from build123d import *

# Parameters (mm, degrees)
SKETCH_1_R          = 62.5
SKETCH_1_R_2        = 40.5
SKETCH_1_R_3        = 2.25
SKETCH_1_R_4        = 1.9
EXTRUDE_1_DEPTH     = 11.5
SKETCH_2_R          = 42.625
CUT_EXTRUDE_1_DEPTH = 9.5


with BuildPart() as part:
    # 草图1 → 凸台-拉伸1 (new body)
    with BuildSketch(Plane.XY):
        Circle(SKETCH_1_R)
        Circle(SKETCH_1_R_2, mode=Mode.SUBTRACT)
        with Locations((0, -52.5)):
            Circle(SKETCH_1_R_3, mode=Mode.SUBTRACT)
        with Locations((-28.383642916, -44.165810474)):
            Circle(SKETCH_1_R_3, mode=Mode.SUBTRACT)
        with Locations((-47.755679756, -21.809288183)):
            Circle(SKETCH_1_R_3, mode=Mode.SUBTRACT)
        with Locations((-51.965625699, 7.471529009)):
            Circle(SKETCH_1_R_3, mode=Mode.SUBTRACT)
        with Locations((-39.676852654, 34.380188532)):
            Circle(SKETCH_1_R_3, mode=Mode.SUBTRACT)
        with Locations((-14.790959234, 50.373381115)):
            Circle(SKETCH_1_R_3, mode=Mode.SUBTRACT)
        with Locations((14.790959234, 50.373381115)):
            Circle(SKETCH_1_R_3, mode=Mode.SUBTRACT)
        with Locations((39.676852654, 34.380188532)):
            Circle(SKETCH_1_R_3, mode=Mode.SUBTRACT)
        with Locations((51.965625699, 7.471529009)):
            Circle(SKETCH_1_R_3, mode=Mode.SUBTRACT)
        with Locations((47.755679756, -21.809288183)):
            Circle(SKETCH_1_R_3, mode=Mode.SUBTRACT)
        with Locations((28.383642916, -44.165810474)):
            Circle(SKETCH_1_R_3, mode=Mode.SUBTRACT)
        with Locations((-44.2113501, -38.309352936)):
            Circle(SKETCH_1_R_4, mode=Mode.SUBTRACT)
        with Locations((-57.90455435, -8.325418039)):
            Circle(SKETCH_1_R_4, mode=Mode.SUBTRACT)
        with Locations((-53.213471728, 24.301778261)):
            Circle(SKETCH_1_R_4, mode=Mode.SUBTRACT)
        with Locations((-31.627487821, 49.213331671)):
            Circle(SKETCH_1_R_4, mode=Mode.SUBTRACT)
        with Locations((0, 58.5)):
            Circle(SKETCH_1_R_4, mode=Mode.SUBTRACT)
        with Locations((31.627487821, 49.213331671)):
            Circle(SKETCH_1_R_4, mode=Mode.SUBTRACT)
        with Locations((53.213471728, 24.301778261)):
            Circle(SKETCH_1_R_4, mode=Mode.SUBTRACT)
        with Locations((57.90455435, -8.325418039)):
            Circle(SKETCH_1_R_4, mode=Mode.SUBTRACT)
        with Locations((44.2113501, -38.309352936)):
            Circle(SKETCH_1_R_4, mode=Mode.SUBTRACT)
        with Locations((16.481354575, -56.130338956)):
            Circle(SKETCH_1_R_4, mode=Mode.SUBTRACT)
        with Locations((-16.481354575, -56.130338956)):
            Circle(SKETCH_1_R_4, mode=Mode.SUBTRACT)
    extrude(amount=EXTRUDE_1_DEPTH)

    # 草图2 → 切除-拉伸1 (cut)
    with BuildSketch(Plane.XY.offset(11.5)):
        Circle(SKETCH_2_R)
    extrude(amount=-CUT_EXTRUDE_1_DEPTH, mode=Mode.SUBTRACT)


solid = part.part
Check sheet for the modelled part. Datum: model origin and axes. Units: mm. A direction names the side the tool comes from. Coordinates: 2 decimals unless noted, no trailing zeros. Write each loop counter-clockwise with the first axis right and the second up, starting at its lowest first coordinate (ties: lowest second). Pieces come first, ordered by that corner, then holes.
Item 1: Depth check by flat-ended pin: pin 1 Ø3 at (x, y) = (-44.21, -38.31) entering from -Z; pin 2 Ø3 at (y, z) = (3, 3) entering from +X; pin 3 Ø5 at (x, z) = (-49, 2.5) entering from +Y; pin 4 Ø5 at (x, z) = (11.5, 8.5) entering from +Y. Enter the tip coordinate at first touch or a pass-through.
Numbers:
pin 1: passes through
pin 2: stops at x = 62.48
pin 3: stops at y = 41.76
pin 4: stops at y = 61.85
Item 2: Cross-section at B-B on x = -36. Record the boundary of the cut face in (y, z), then the cut area to 3 significant figures.
Numbers:
outline: (-51.09, 0) - (-18.55, 0) - (-18.55, 2) - (-22.82, 2) - (-22.82, 11.5) - (-51.09, 11.5) - close; (18.55, 0) - (51.09, 0) - (51.09, 11.5) - (22.82, 11.5) - (22.82, 2) - (18.55, 2) - close
area: 667 mm2
Item 3: Scan lines: probe 1 along Y at (x, z) = (0, 6.75) (3 decimals); probe 2 along Y at (x, z) = (28, 9.5); probe 3 along Y at (x, z) = (-16, 10.5). Record each from-to range of solid material in increasing order.
Numbers:
probe 1: y = -62.5 to -54.75, -50.25 to -42.625, 42.625 to 56.6, 60.4 to 62.5
probe 2: y = -55.88 to -46.38, -41.95 to -32.14, 32.14 to 55.88
probe 3: y = -60.42 to -57.97, -54.29 to -39.51, 39.51 to 48.48, 52.27 to 60.42
Item 4: Access from +Z, -Z, +X, -X, +Y, -Y to the whole of each face (thin tool, end or side, straight path). Record for faces 1 (the face through (16, -38, 2)), 2 (the face through (-59.8, -8.2, 5.7)).
Numbers:
face 1: +Z
face 2: +Z, -Z
Item 5: Cross-section at C-C on z = 8.75. Count the separate pieces of the cut face and the enclosed holes in it, then the cut area to 3 significant figures.
Numbers:
separate pieces: 1
enclosed holes: 23
area: 6,260 mm2
Item 6: Cross-section at A-A on y = 0. Record the boundary of the cut face in (x, z) (3 decimals).
Numbers:
outline: (-62.5, 0) - (-40.5, 0) - (-40.5, 2) - (-42.625, 2) - (-42.625, 11.5) - (-62.5, 11.5) - close; (40.5, 0) - (62.5, 0) - (62.5, 11.5) - (42.625, 11.5) - (42.625, 2) - (40.5, 2) - close
Item 7: Cross-section at D-D on y = 58.5. Record the boundary of the cut face in (x, z), then the cut area to 3 significant figures.
Numbers:
outline: (-22, 0) - (-1.9, 0) - (-1.9, 11.5) - (-22, 11.5) - close; (1.9, 0) - (22, 0) - (22, 11.5) - (1.9, 11.5) - close
area: 462 mm2
